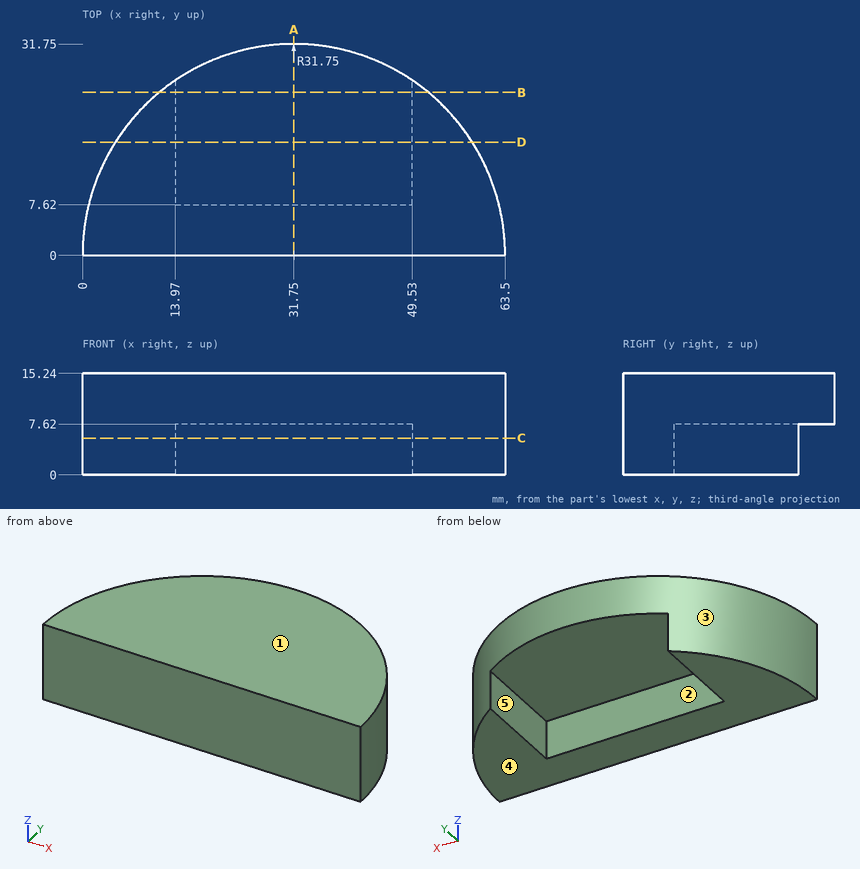
For this review, use the dimensioned drawing (mm, ordinates from the lowest corner) and the shaded views. A direction names the side the tool comes from. Coordinates: 2 decimals unless noted, no trailing zeros. Loops run counter-clockwise (first coordinate to the right, second up) from the corner with the lowest first, then second, coordinate; pieces in that order, holes last. Notation, with made-up numbers: (54, -5.5) - (82, -5.5) arc R30 cw to (82, 24.5) - close; hole circle Ø8 at (-9.5, 1.25). An arc over 180 degrees is marked (long way). Use CSV: the item, a comma, the result in double quotes. Start each with the question number.
1) The part is to be moulded in two halves that separate along X. For the marked faces 1, 2 and 3, say which applies: +X half, -X half, draft (parallel to the pull), parting line (faces both ways), or undercut.
2) Tool access review of the marked faces 4 and 5: name each direction out of +Z, -Z, +X, -X, +Y, -Y from which nothing blocks a thin tool from reaching the whole face with its end or side.
3) For pin 1 Ø4 at (x, z) = (7, 8) entering from +Y; pin 2 Ø2.5 at (y, z) = (13, 4) entering from +X; pin 3 Ø2.5 at (x, z) = (38, 3) entering from +Y, all flat-tipped, find the tip position at first contact; note any pin that passes through.
4) Wall thickness on L1, parallel to Z at x = 17.5, y = 21; L2, parallel to Y at x = 36.5, z = 7; L3, parallel to X at y = 9, z = 1.25: over which ranges is each line inside the solid? List them lowest first. Write a range as from..to.
5) Consider section A-A on x = 31.75. Write out the cut boundary in (y, z).
6) Consider section D-D on y = 17. Write out the cut boundary in (x, z), then the cut area to 3 significant figures.
7) Consider section B-B on y = 24.5. Write out the cut boundary in (x, z), then the cut area to 3 significant figures.
8) Consider section C-C on z = 5.5. Write out the cut boundary in (x, y), then the cut area to 3 significant figures.
Geometry says:
1,face 1,"draft"
1,face 2,"undercut"
1,face 3,"parting line"
2,face 4,"-Z, +X, -X, +Y, -Y"
2,face 5,"-Z, +Y"
3,pin 1,"y = 22.15"
3,pin 2,"x = 61.25"
3,pin 3,"y = 7.62"
4,L1,"7.62..15.24"
4,L2,"0..7.62"
4,L3,"1.3..13.97, 49.53..62.2"
5,outline,"(0, 0) - (7.62, 0) - (7.62, 7.62) - (31.75, 7.62) - (31.75, 15.24) - (0, 15.24) - close"
6,outline,"(4.93, 0) - (13.97, 0) - (13.97, 7.62) - (49.53, 7.62) - (49.53, 0) - (58.57, 0) - (58.57, 15.24) - (4.93, 15.24) - close"
6,area,"546 mm^2"
7,outline,"(11.56, 0) - (13.97, 0) - (13.97, 7.62) - (49.53, 7.62) - (49.53, 0) - (51.94, 0) - (51.94, 15.24) - (11.56, 15.24) - close"
7,area,"345 mm^2"
8,outline,"(0, 0) - (63.5, 0) arc R31.75 ccw to (49.53, 26.3) - (49.53, 7.62) - (13.97, 7.62) - (13.97, 26.3) arc R31.75 ccw to start"
8,area,"788 mm^2"
